Could you check a few things on this model? Use its own coordinates, in mm. Face numbers are marked on the shaded views. A direction names the side the tool comes from. Give positions to 0.01 mm unless a question says otherwise; leave off trailing zeros. Loops run counter-clockwise (first coordinate to the right, second up) from the corner with the lowest first, then second, coordinate; pieces in that order, holes last. Notation, with made-up numbers: (-4.5, 32.25) - (2.5, 32.25) arc R15 ccw to (2.5, 60.25) - close; hole circle Ø10 at (71, -30.75). An arc over 180 degrees is marked (long way). Use CSV: the item, a comma, the result in double quotes.
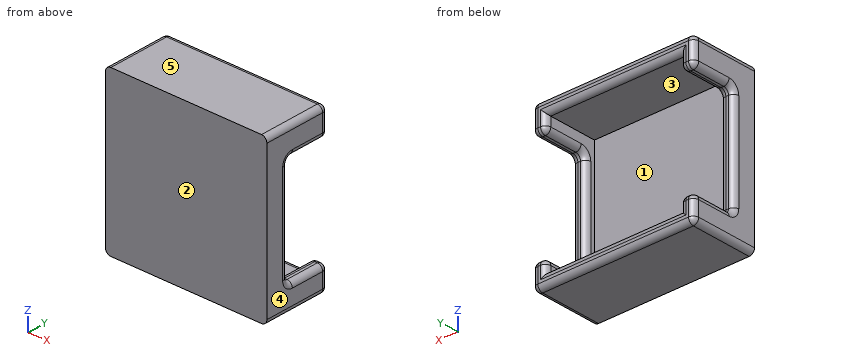
from build123d import *

# Parameters (mm, degrees)
SKETCH5_W           = 60
SKETCH5_H           = 60
BOSS_EXTRUDE3_DEPTH = 25
SHELL1_T            = -5
SKETCH6_W           = 40
SKETCH6_H           = 50
CUT_EXTRUDE2_DEPTH  = 100
FILLET2_R           = 2


with BuildPart() as part:
    # Sketch5 → Boss-Extrude3 (new body)
    with BuildSketch(Plane(origin=(0, 0, 0), x_dir=(1, 0, 0), z_dir=(0, 1, 0))):
        Rectangle(SKETCH5_W, SKETCH5_H)
    extrude(amount=BOSS_EXTRUDE3_DEPTH)

    # Shell1
    shell1_openings = [part.faces().sort_by_distance(p)[0] for p in [
        (0, 25, 0),
    ]]
    offset(amount=SHELL1_T, openings=shell1_openings, kind=Kind.INTERSECTION)

    # Sketch6 → Cut-Extrude2 (cut)
    with BuildSketch(Plane(origin=(30, 0, 0), x_dir=(0, 0, -1), z_dir=(1, 0, 0))):
        with Locations((0.42294972, 33.504960927)):
            Rectangle(SKETCH6_W, SKETCH6_H)
    extrude(amount=-CUT_EXTRUDE2_DEPTH, mode=Mode.SUBTRACT)

    # Fillet2
    fillet2_edges = [part.edges().sort_by_distance(p)[0] for p in [
        (-30, 25, -25.21147486),
        (25, 25, 22.28852514),
        (0, 25, -25),
        (-25, 25, -22.71147486),
        (0, 25, 30),
        (0, 25, 25),
        (-25, 25, 22.28852514),
        (-25, 16.752480464, 19.57705028),
        (-25, 8.504960927, -0.42294972),
        (-25, 16.752480464, -20.42294972),
        (25, 25, -22.71147486),
        (-30, 25, 24.78852514),
        (30, 25, -25.21147486),
        (30, 16.752480464, -20.42294972),
        (30, 16.752480464, 19.57705028),
        (30, 8.504960927, -0.42294972),
        (27.5, 25, -20.42294972),
        (-30, 16.752480464, -20.42294972),
        (-27.5, 25, -20.42294972),
        (-30, 8.504960927, -0.42294972),
        (-27.5, 8.504960927, -20.42294972),
        (25, 8.504960927, -0.42294972),
        (27.5, 8.504960927, -20.42294972),
        (27.5, 25, 19.57705028),
        (27.5, 8.504960927, 19.57705028),
        (-27.5, 25, 19.57705028),
        (-30, 16.752480464, 19.57705028),
        (-27.5, 8.504960927, 19.57705028),
        (25, 16.752480464, -20.42294972),
        (25, 16.752480464, 19.57705028),
        (30, 25, 24.78852514),
        (30, 12.5, 30),
        (-30, 12.5, 30),
        (-30, 12.5, -30),
        (30, 12.5, -30),
        (0, 25, -30),
    ]]
    fillet(fillet2_edges, radius=FILLET2_R)


solid = part.part
1) We'd pull the mould along Z, two halves only. Please class the marked faces 3, 4 and 5: +Z half, -Z half, draft (parallel to the pull), parting line (faces both ways), or undercut.
Answer below:
face 3,"undercut"
face 4,"draft"
face 5,"+Z half"
2) Which directions (+Z, -Z, +X, -X, +Y, -Y) give clear straight access to the entire face, cutting with the end or side of a thin tool? Please do the marked faces 1 and 2.
Answer below:
face 1,"+Y"
face 2,"+Z, -Z, +X, -X, -Y"
3) Suppose I cut it at C-C (x = -7). Please give me the cut outline in (y, z), plus the area to 3 significant figures.
Answer below:
outline,"(0, -30) - (23, -30) arc R2 ccw to (25, -28) - (25, -27) arc R2 ccw to (23, -25) - (5, -25) - (5, 25) - (23, 25) arc R2 ccw to (25, 27) - (25, 28) arc R2 ccw to (23, 30) - (0, 30) - close"
area,"497 mm2"
4) I'm going to push flat-ended pins straight in: P1, Ø8, axis at x = -2.5, z = -15.5, coming from the +Y side; P2, Ø9, axis at y = 12.5, z = -12, coming from the -X side; P3, Ø5.5, axis at y = 11, z = 6, coming from the +X side. Where does each tip first touch, or does it pass through?
Answer below:
P1,"stops at y = 5"
P2,"stops at x = -29.33"
P3,"stops at x = 28.98"
5) Suppose I cut it at A-A (y = 12.25). Please give me the cut outline in (x, z), plus the area to 3 significant figures.
Answer below:
outline,"(-30, -28) arc R2 ccw to (-28, -30) - (28, -30) arc R2 ccw to (30, -28) - (30, -22.42) arc R2 ccw to (28, -20.42) - (27, -20.42) arc R2 ccw to (25, -22.42) - (25, -25) - (-25, -25) - (-25, -22.42) arc R2 ccw to (-27, -20.42) - (-28, -20.42) arc R2 ccw to (-30, -22.42) - close; (-30, 21.58) arc R2 ccw to (-28, 19.58) - (-27, 19.58) arc R2 ccw to (-25, 21.58) - (-25, 25) - (25, 25) - (25, 21.58) arc R2 ccw to (27, 19.58) - (28, 19.58) arc R2 ccw to (30, 21.58) - (30, 28) arc R2 ccw to (28, 30) - (-28, 30) arc R2 ccw to (-30, 28) - close"
area,"690 mm2"
6) Suppose I cut it at B-B (z = 11). Please give me the cut outline in (x, y).
Answer below:
outline,"(-30, 0) - (30, 0) - (30, 6.5) arc R2 ccw to (28, 8.5) - (27, 8.5) arc R2 ccw to (25, 6.5) - (25, 5) - (-25, 5) - (-25, 6.5) arc R2 ccw to (-27, 8.5) - (-28, 8.5) arc R2 ccw to (-30, 6.5) - close"
7) I need wall thicknesses on line 1 along Z through (x, y) = (11.5, 6.5); line 2 along Y through (x, z) = (9.5, -19); line 3 along X through (y, z) = (7.75, -16.5). Which ranges of each line are inside material? Lowest first, please.
Answer below:
line 1,"z = -30 to -25, 25 to 30"
line 2,"y = 0 to 5"
line 3,"x = -29.57 to -25.43, 25.43 to 29.57"
